Job drawing, mm, ordinate dimensions from the low corner. One solid piece. Give positions to 0.01 mm unless a question says otherwise; leave off trailing zeros. Order: outer loops, then holes, each group sorted by start corner. A loop starts at its lowest first (then second) coordinate and runs counter-clockwise, first axis right, second up. Notation, with made-up numbers: M -28.75,-4.75 L 29.25,-4.75 A31 ccw 29.25,33.25 Z; hole C 15,52.5 d7. An arc over 180 degrees is marked long. Put each result on its own line as item: value. Start each with the question number.
1) Cut at B-B (z = 87.5). Write the cut outline in (x, y), and give its area (3 significant figures).
2) Cut at C-C (x = 26). Write the cut outline in (y, z).
3) Drill centre lines: line 1 (X direction, y = 7.7, z = 2.55) (3 decimals); line 2 (X direction, y = 8.75, z = 32); line 3 (Y direction, x = 40.65, z = 2.8) (3 decimals). Where is each one in solid material? Low to high. Write a range as [from, to].
4) Pin check, flat tips, straight feed: pin 1 (8 mm diameter, centred on x = 63, y = 8, fed in from -Z); pin 2 (1.6 mm diameter, centred on x = 36, y = 1, fed in from +Z); pin 3 (1.6 mm diameter, centred on x = 41.5, y = 6.5, fed in from +Z). Stop position of each tip, or through.
5) Cut at A-A (x = 40.65). Write the cut outline in (y, z) (3 decimals).
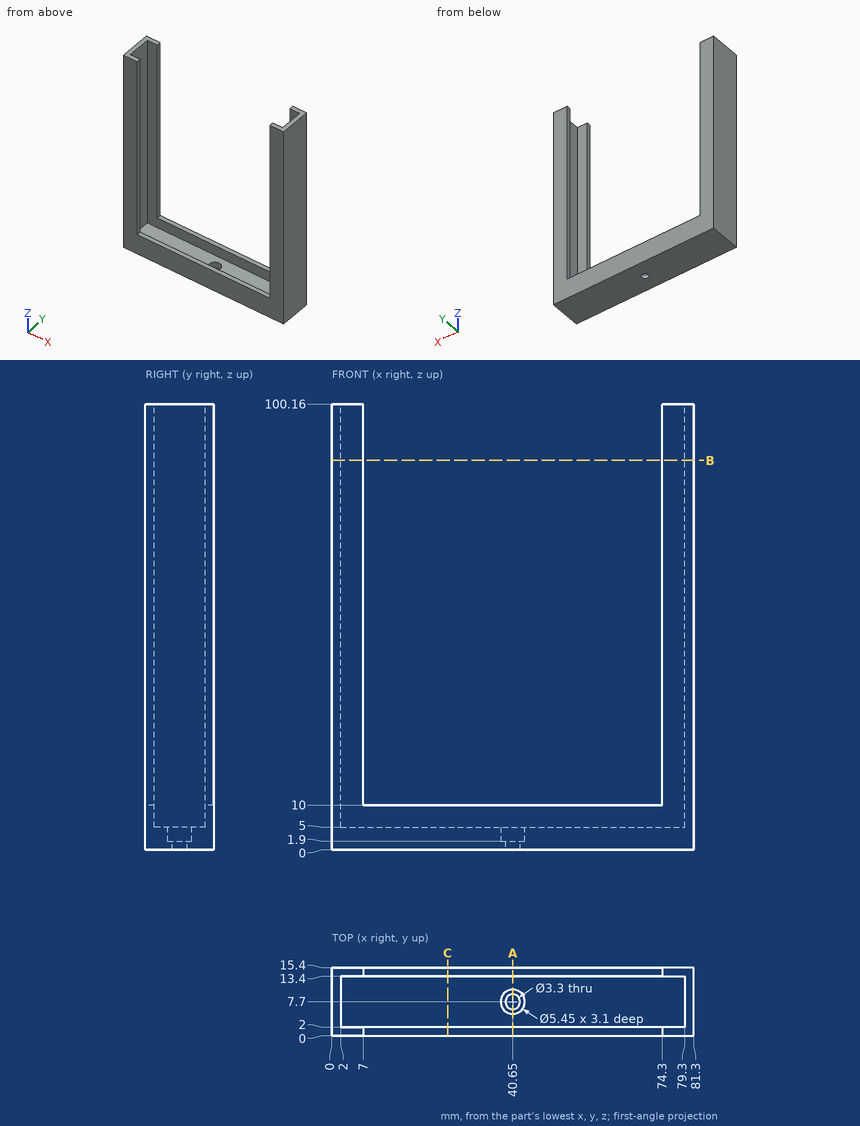
Solution:
1. outline: M 0,0 L 7,0 L 7,2 L 2,2 L 2,13.4 L 7,13.4 L 7,15.4 L 0,15.4 Z; M 74.3,0 L 81.3,0 L 81.3,15.4 L 74.3,15.4 L 74.3,13.4 L 79.3,13.4 L 79.3,2 L 74.3,2 Z
1. area: 102 mm²
2. outline: M 0,0 L 15.4,0 L 15.4,10 L 13.4,10 L 13.4,5 L 2,5 L 2,10 L 0,10 Z
3. line 1: [0, 37.925], [43.375, 81.3]
3. line 2: [0, 2], [79.3, 81.3]
3. line 3: [0, 4.975], [10.425, 15.4]
4. pin 1: z = 0
4. pin 2: z = 10
4. pin 3: z = 1.9
5. outline: M 0,0 L 6.05,0 L 6.05,1.9 L 4.975,1.9 L 4.975,5 L 2,5 L 2,10 L 0,10 Z; M 9.35,0 L 15.4,0 L 15.4,10 L 13.4,10 L 13.4,5 L 10.425,5 L 10.425,1.9 L 9.35,1.9 Z
